from build123d import *

# Parameters (mm, degrees)
SKETCH1_W           = 34.925
SKETCH1_H           = 34.925
SKETCH1_W_2         = 30.9626
SKETCH1_H_2         = 30.9626
BOSS_EXTRUDE1_DEPTH = 165.1
SKETCH2_W           = 6.550000108
SKETCH2_H           = 44.650000108
CUT_EXTRUDE1_DEPTH  = 170.654662569


with BuildPart() as part:
    # Sketch1 → Boss-Extrude1 (new, symmetric)
    with BuildSketch(Plane(origin=(0, 0, 0), x_dir=(1, 0, 0), z_dir=(0, 1, 0))):
        Rectangle(SKETCH1_W, SKETCH1_H)
        Rectangle(SKETCH1_W_2, SKETCH1_H_2, mode=Mode.SUBTRACT)
    extrude(amount=BOSS_EXTRUDE1_DEPTH, both=True)

    # Sketch2 → Cut-Extrude1 (cut, through all)
    with BuildSketch(Plane(origin=(17.4625, 0, 0), x_dir=(0, 0, -1), z_dir=(1, 0, 0))):
        with Locations((0, 63.5)):
            Rectangle(SKETCH2_W, SKETCH2_H)
    extrude(amount=-CUT_EXTRUDE1_DEPTH, mode=Mode.SUBTRACT)


solid = part.part
CAD build for the part. Positions are in the model's coordinates, mm. A direction names the side the tool comes from. Coordinates: 2 decimals unless noted, no trailing zeros. Loops run counter-clockwise (first coordinate to the right, second up) from the corner with the lowest first, then second, coordinate; pieces in that order, holes last. Notation, with made-up numbers: (21.25, 41.25) -> (68.25, 41.25) arc R24 ccw to (68.25, 64.25) -> close; hole circle Ø11 at (66.5, 15). An arc over 180 degrees is marked (long way). One line per item, written item: value.
1. Slice it at A-A on z = 11. Write the cut outline in (x, y).
Answers:
outline: (-17.46, -165.1) -> (-15.48, -165.1) -> (-15.48, 165.1) -> (-17.46, 165.1) -> close; (15.48, -165.1) -> (17.46, -165.1) -> (17.46, 165.1) -> (15.48, 165.1) -> close
2. Slice it at B-B on x = -6. Write the cut outline in (y, z).
Answers:
outline: (-165.1, -17.46) -> (165.1, -17.46) -> (165.1, -15.48) -> (-165.1, -15.48) -> close; (-165.1, 15.48) -> (165.1, 15.48) -> (165.1, 17.46) -> (-165.1, 17.46) -> close
3. Flat gauge pin, fed straight in: P1, Ø12, axis at x = 3.5, z = 12, coming from the +Y side. Where does the tip first touch, or does it go through?
Answers:
P1: stops at y = 165.1
4. Drill centre lines: line 1 (X direction, y = 144.5, z = -5); line 2 (Y direction, x = -16, z = -2) (3 decimals). Where is each one in solid material? Low to high. Write a range as [from, to].
Answers:
line 1: x = [-17.46, -15.48], [15.48, 17.46]
line 2: y = [-165.1, 41.175], [85.825, 165.1]
5. Pull direction Z, two halves, no side cores. Call faces 3 (the face through (15.481, 2, 0)), 4 (the face through (17.462, 2, 0)), 5 (the face through (0, 2, -17.462)): pulls with the +Z half, pulls with the -Z half, needs draft (parallel to the pull), parting line crosses it, or undercut.
Answers:
face 3: undercut
face 4: needs draft
face 5: pulls with the -Z half
6. Slice it at C-C on y = -111. Write the cut outline in (x, z), and give its area (3 significant figures).
Answers:
outline: (-17.46, -17.46) -> (17.46, -17.46) -> (17.46, 17.46) -> (-17.46, 17.46) -> close; hole (-15.48, -15.48) -> (15.48, -15.48) -> (15.48, 15.48) -> (-15.48, 15.48) -> close
area: 261 mm^2
7. Which spindle directions (+Z, -Z, +X, -X, +Y, -Y) get a long thin tool onto all of the face, cutting with end or side? Do faces 1 (the face through (0, 2, 17.462)), 2 (the face through (-15.481, 2, 0)). Say none if no direction does.
Answers:
face 1: +Z, +X, -X, +Y, -Y
face 2: +Y, -Y
